Check sheet for the modelled part. Datum: model origin and axes. Units: mm. Face numbers are marked on the shaded views. A direction names the side the tool comes from. Give positions to 0.01 mm unless a question says otherwise; leave off trailing zeros. Write each loop counter-clockwise with the first axis right and the second up, starting at its lowest first coordinate (ties: lowest second). Pieces come first, ordered by that corner, then holes. Notation, with made-up numbers: (51.25, 84) -> (106.25, 84) arc R34 cw to (106.25, 119) -> close; hole circle Ø11 at (53.5, 11). An arc over 180 degrees is marked (long way). Use a Markdown table: item, result. Add a question column.
1. Scan line: probe 1 along X at (y, z) = (12.5, 10). Record every from-to range of solid material in increasing order. Write a range as [from, to].
2. Cross-section at A-A (x = -14). Enter the section's corners in (y, z), then the cut area to 3 significant figures.
3. Gauge pin test, flat ends, axial feed: P1, Ø7.5, axis at x = -12, z = 12.5, coming from the +Y side; P2, Ø20, axis at y = 14.5, z = 10, coming from the -X side; P3, Ø2, axis at x = 16.5, z = 10.5, coming from the -Y side. Record the tip position at first contact, or that the pin passes through.
4. Set-up check for the marked faces 1, 2 and 3: record each of +Z, -Z, +X, -X, +Y, -Y from which the full face is reachable in a straight line by a thin tool's end or side.
5. Cross-section at B-B (z = 18.5). Enter the section's corners in (x, y), then the cut area to 3 significant figures.
from build123d import *

# Parameters (mm, degrees)
F0_W     = 2
F0_H     = 55
F1_DEPTH = 38
F7_COUNT = 4
F9_SIZE  = 0.7


with BuildPart() as f1:
    # F0 (on Top) → F1 (new body)
    with BuildSketch(Plane.XY):
        with Locations((-1, 27.5)):
            Rectangle(F0_W, F0_H)
    extrude(amount=F1_DEPTH)


with BuildPart() as f1_1:
    # F3: moved
    add(f1.part.moved(Location((1, 0, 0))))


with BuildPart() as f1_2:
    # F5: moved
    add(f1_1.part.moved(Location((0, -27.5, 0))))


with BuildPart() as f7_1:
    # F7: instance of F1
    add(f1_2.part.rotate(Axis((0, 0, 29.2499251664), (0, 0, 1)), 1 * 360 / F7_COUNT))


with BuildPart() as f7_2:
    # F7: instance of F1
    add(f1_2.part.rotate(Axis((0, 0, 29.2499251664), (0, 0, 1)), 2 * 360 / F7_COUNT))


with BuildPart() as f7_3:
    # F7: instance of F1
    add(f1_2.part.rotate(Axis((0, 0, 29.2499251664), (0, 0, 1)), 3 * 360 / F7_COUNT))


with BuildPart() as f1_3:
    add(f1_2.part)

    # F8: union F7_1, F7_2, F7_3
    add(f7_1.part)
    add(f7_2.part)
    add(f7_3.part)

    # F9
    f9_edges = [f1_3.edges().sort_by_distance(p)[0] for p in [
        (14.25, 1, 0),
        (1, 1, 19),
        (14.25, 1, 38),
        (27.5, 1, 19),
        (1, 14.25, 0),
        (1, 27.5, 19),
        (1, 14.25, 38),
        (-14.25, 1, 0),
        (-27.5, 1, 19),
        (-14.25, 1, 38),
        (-1, 1, 19),
        (-1, 14.25, 0),
        (-1, 14.25, 38),
        (-1, 27.5, 19),
        (-1, -14.25, 0),
        (-1, -27.5, 19),
        (-1, -14.25, 38),
        (-1, -1, 19),
        (-14.25, -1, 0),
        (-14.25, -1, 38),
        (-27.5, -1, 19),
        (1, -14.25, 0),
        (1, -1, 19),
        (1, -14.25, 38),
        (1, -27.5, 19),
        (14.25, -1, 0),
        (27.5, -1, 19),
        (14.25, -1, 38),
    ]]
    chamfer(f9_edges, length=F9_SIZE)


solid = f1_3.part
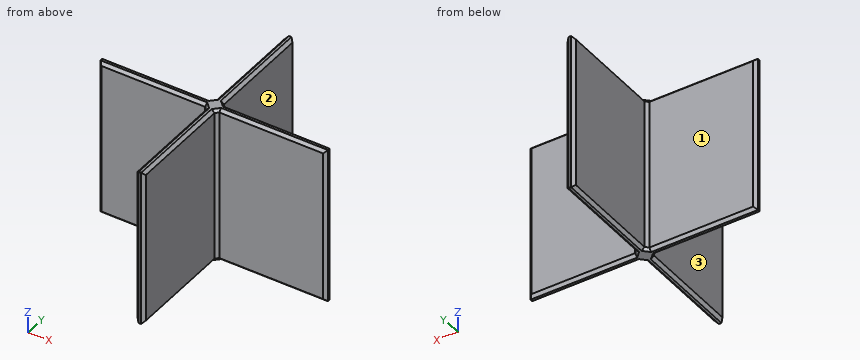
Worked answers:
| question | item | result |
|---|---|---|
| 1 | probe 1 | x = [-1, 1] |
| 2 | outline | (-1, 0.7) -> (-0.3, 0) -> (0.3, 0) -> (1, 0.7) -> (1, 37.3) -> (0.3, 38) -> (-0.3, 38) -> (-1, 37.3) -> close |
| 2 | area | 75.0 mm² |
| 3 | P1 | stops at y = 1 |
| 3 | P2 | stops at x = -1 |
| 3 | P3 | stops at y = -1 |
| 4 | face 1 | +Z, -Z, -X, +Y |
| 4 | face 2 | +Z, -Z, +X, +Y |
| 4 | face 3 | +Z, -Z, -X, -Y |
| 5 | outline | (-27.5, -0.3) -> (-26.8, -1) -> (-1.7, -1) -> (-1, -1.7) -> (-1, -26.8) -> (-0.3, -27.5) -> (0.3, -27.5) -> (1, -26.8) -> (1, -1.7) -> (1.7, -1) -> (26.8, -1) -> (27.5, -0.3) -> (27.5, 0.3) -> (26.8, 1) -> (1.7, 1) -> (1, 1.7) -> (1, 26.8) -> (0.3, 27.5) -> (-0.3, 27.5) -> (-1, 26.8) -> (-1, 1.7) -> (-1.7, 1) -> (-26.8, 1) -> (-27.5, 0.3) -> close |
| 5 | area | 215 mm² |
